The listing builds one solid part. Answer for the finished solid, in the listing's coordinates (mm). Give positions to 0.01 mm unless a question says otherwise; leave off trailing zeros. Order: outer loops, then holes, each group sorted by start corner. A loop starts at its lowest first (then second) coordinate and runs counter-clockwise, first axis right, second up. Notation, with made-up numbers: (28, -6.75) - (84, -6.75) arc R11 cw to (84, 1.25) - close; hole circle Ø1 at (67, 47). An arc over 180 degrees is marked (long way). Write each question's results on one line, items separated by ' | '. Start each with the question number.
1. Find the intervals of material crossed by L1, parallel to Z at x = -10, y = 5.25; L2, parallel to X at y = 1.5, z = -24; L3, parallel to Z at x = -13.5, y = 4, in increasing order.
2. Section B-B (x = -13) is taken. Give the vertices of the cut face in (y, z) (3 decimals).
3. Flat-ended cylindrical pins translate along their axes: pin 1 (2.5 mm diameter, centred on y = 3.5, z = 23.5, fed in from +X); pin 2 (5 mm diameter, centred on y = 8, z = -24, fed in from +X); pin 3 (0.9 mm diameter, centred on x = 10.5, y = 2.5, fed in from +Z); pin 4 (2 mm diameter, centred on x = 8.5, z = -7, fed in from -Y). Find the tip coordinate at first contact, or state that the pin passes through.
4. Section C-C (z = 23.5) is taken. Give the vertices of the cut face in (x, y) (3 decimals), and give its area (3 significant figures).
5. Section D-D (x = -20.5) is taken. Give the vertices of the cut face in (y, z) (3 decimals), and give its area (3 significant figures).
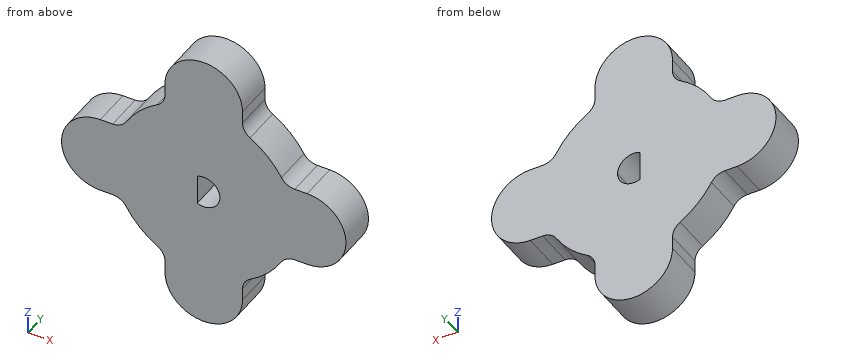
from build123d import *

# Parameters (mm, degrees)
SKETCH1_W           = 19.05
SKETCH1_H           = 19.05
BOSS_EXTRUDE1_DEPTH = 9.525
FILLET1_R           = 3.81
CUT_EXTRUDE1_DEPTH  = 61.38309394


with BuildPart() as part:
    # Sketch1 → Boss-Extrude1 (new body)
    with BuildSketch(Plane(origin=(0, 0, 0), x_dir=(1, 0, 0), z_dir=(0, 1, 0))):
        with BuildLine():
            Line((-3.432814358, 26.008484179), (-22.482814358, 26.008484179))
            Line((-22.482814358, 26.008484179), (-22.482814358, 20.688947321))
            ThreePointArc((-22.482814358, 20.688947321), (-12.957814358, 22.833484179), (-3.432814358, 20.688947321))
            Line((-3.432814358, 20.688947321), (-3.432814358, 26.008484179))
        make_face()
        with BuildLine():
            ThreePointArc((-3.432814358, 20.688947321), (-12.957814358, 22.833484179), (-22.482814358, 20.688947321))
            Line((-22.482814358, 20.688947321), (-22.482814358, 10.133484179))
            Line((-22.482814358, 10.133484179), (-3.432814358, 10.133484179))
            Line((-3.432814358, 10.133484179), (-3.432814358, 20.688947321))
        make_face()
        with BuildLine():
            ThreePointArc((-22.482814358, 26.008484179), (-12.957814358, 35.533484179), (-3.432814358, 26.008484179))
            Line((-3.432814358, 26.008484179), (-22.482814358, 26.008484179))
        make_face()
        with Locations((-12.957814358, 0.608484179)):
            Rectangle(SKETCH1_W, SKETCH1_H)
        with BuildLine():
            Line((-22.482814358, -8.916515821), (-22.482814358, 10.133484179))
            Line((-22.482814358, 10.133484179), (-33.0382775, 10.133484179))
            ThreePointArc((-33.0382775, 10.133484179), (-35.182814358, 0.608484179), (-33.0382775, -8.916515821))
            Line((-33.0382775, -8.916515821), (-22.482814358, -8.916515821))
        make_face()
        with BuildLine():
            ThreePointArc((-33.0382775, -8.916515821), (-35.182814358, 0.608484179), (-33.0382775, 10.133484179))
            Line((-33.0382775, 10.133484179), (-38.357814358, 10.133484179))
            Line((-38.357814358, 10.133484179), (-38.357814358, -8.916515821))
            Line((-38.357814358, -8.916515821), (-33.0382775, -8.916515821))
        make_face()
        with BuildLine():
            Line((-38.357814358, 10.133484179), (-38.357814358, -8.916515821))
            ThreePointArc((-38.357814358, -8.916515821), (-47.882814358, 0.608484179), (-38.357814358, 10.133484179))
        make_face()
        with BuildLine():
            Line((-22.482814358, -19.471978963), (-22.482814358, -8.916515821))
            Line((-22.482814358, -8.916515821), (-33.0382775, -8.916515821))
            ThreePointArc((-33.0382775, -8.916515821), (-28.67326257, -15.106964033), (-22.482814358, -19.471978963))
        make_face()
        with BuildLine():
            Line((-3.432814358, -8.916515821), (-22.482814358, -8.916515821))
            Line((-22.482814358, -8.916515821), (-22.482814358, -19.471978963))
            ThreePointArc((-22.482814358, -19.471978963), (-12.957814358, -21.616515821), (-3.432814358, -19.471978963))
            Line((-3.432814358, -19.471978963), (-3.432814358, -8.916515821))
        make_face()
        with BuildLine():
            ThreePointArc((-3.432814358, -19.471978963), (-12.957814358, -21.616515821), (-22.482814358, -19.471978963))
            Line((-22.482814358, -19.471978963), (-22.482814358, -24.791515821))
            Line((-22.482814358, -24.791515821), (-3.432814358, -24.791515821))
            Line((-3.432814358, -24.791515821), (-3.432814358, -19.471978963))
        make_face()
        with BuildLine():
            ThreePointArc((-3.432814358, -24.791515821), (-12.957814358, -34.316515821), (-22.482814358, -24.791515821))
            Line((-22.482814358, -24.791515821), (-3.432814358, -24.791515821))
        make_face()
        with BuildLine():
            ThreePointArc((7.122648784, 10.133484179), (2.757633854, 16.323932391), (-3.432814358, 20.688947321))
            Line((-3.432814358, 20.688947321), (-3.432814358, 10.133484179))
            Line((-3.432814358, 10.133484179), (7.122648784, 10.133484179))
        make_face()
        with BuildLine():
            Line((7.122648784, 10.133484179), (-3.432814358, 10.133484179))
            Line((-3.432814358, 10.133484179), (-3.432814358, -8.916515821))
            Line((-3.432814358, -8.916515821), (7.122648784, -8.916515821))
            ThreePointArc((7.122648784, -8.916515821), (8.724423976, -4.273233329), (9.267185642, 0.608484179))
            ThreePointArc((9.267185642, 0.608484179), (8.724423976, 5.490201688), (7.122648784, 10.133484179))
        make_face()
        with BuildLine():
            Line((7.122648784, -8.916515821), (-3.432814358, -8.916515821))
            Line((-3.432814358, -8.916515821), (-3.432814358, -19.471978963))
            ThreePointArc((-3.432814358, -19.471978963), (2.757633854, -15.106964033), (7.122648784, -8.916515821))
        make_face()
        with BuildLine():
            Line((12.442185642, 10.133484179), (7.122648784, 10.133484179))
            ThreePointArc((7.122648784, 10.133484179), (8.724423976, 5.490201688), (9.267185642, 0.608484179))
            ThreePointArc((9.267185642, 0.608484179), (8.724423976, -4.273233329), (7.122648784, -8.916515821))
            Line((7.122648784, -8.916515821), (12.442185642, -8.916515821))
            Line((12.442185642, -8.916515821), (12.442185642, 10.133484179))
        make_face()
        with BuildLine():
            ThreePointArc((12.442185642, 10.133484179), (21.967185642, 0.608484179), (12.442185642, -8.916515821))
            Line((12.442185642, -8.916515821), (12.442185642, 10.133484179))
        make_face()
        with BuildLine():
            Line((-22.482814358, 10.133484179), (-22.482814358, 20.688947321))
            ThreePointArc((-22.482814358, 20.688947321), (-28.67326257, 16.323932391), (-33.0382775, 10.133484179))
            Line((-33.0382775, 10.133484179), (-22.482814358, 10.133484179))
        make_face()
    extrude(amount=BOSS_EXTRUDE1_DEPTH)

    # Fillet1
    fillet1_edges = [part.edges().sort_by_distance(p)[0] for p in [
        (-22.482814358, 4.7625, -20.688947321),
        (-3.432814358, 4.7625, -20.688947321),
        (7.122648784, 4.7625, -10.133484179),
        (7.122648784, 4.7625, 8.916515821),
        (-3.432814358, 4.7625, 19.471978963),
        (-22.482814358, 4.7625, 19.471978963),
        (-33.0382775, 4.7625, 8.916515821),
        (-33.0382775, 4.7625, -10.133484179),
    ]]
    fillet(fillet1_edges, radius=FILLET1_R)

    # Sketch2 → Cut-Extrude1 (cut, through all)
    with BuildSketch(Plane(origin=(0, 9.525, 0), x_dir=(1, 0, 0), z_dir=(0, 1, 0))):
        with BuildLine():
            ThreePointArc((-8.989064358, 0.608484179), (-10.784040458, 3.92897866), (-14.545314358, 4.245903637))
            Line((-14.545314358, 4.245903637), (-14.545314358, 0.608484179))
            Line((-14.545314358, 0.608484179), (-8.989064358, 0.608484179))
        make_face()
        with BuildLine():
            Line((-8.989064358, 0.608484179), (-14.545314358, 0.608484179))
            Line((-14.545314358, 0.608484179), (-14.545314358, -3.028935279))
            ThreePointArc((-14.545314358, -3.028935279), (-10.784040458, -2.712010301), (-8.989064358, 0.608484179))
        make_face()
    extrude(amount=-CUT_EXTRUDE1_DEPTH, mode=Mode.SUBTRACT)


solid = part.part
Reported:
1) L1: -35.06 to -3.25, 2.04 to 33.85 | L2: -22.48 to -3.43 | L3: -35.52 to -4.54, 3.32 to 34.3
2) outline: (0, -35.533) - (9.525, -35.533) - (9.525, -4.577) - (0, -4.577) - close; (0, 3.36) - (9.525, 3.36) - (9.525, 34.316) - (0, 34.316) - close
3) pin 1: x = -3.43 | pin 2: x = -3.14 | pin 3: z = 8.92 | pin 4: y = 0
4) outline: (-22.483, 0) - (-3.433, 0) - (-3.433, 9.525) - (-22.483, 9.525) - close | area: 181 mm²
5) outline: (0, -31.826) - (9.525, -31.826) - (9.525, 30.609) - (0, 30.609) - close | area: 595 mm²
